from build123d import *

# Parameters (mm, degrees)
SKETCH_1_W          = 30
SKETCH_1_H          = 20
SKETCH_1_R          = 1.5
EXTRUDE_1_DEPTH     = 3
CUT_EXTRUDE_1_REACH = 20.276
SKETCH_2_R          = 2.5


with BuildPart() as part:
    # 草图1 → 凸台-拉伸1 (new body)
    with BuildSketch(Plane(origin=(0, 0, 0), x_dir=(0, 0, -1), z_dir=(1, 0, 0))):
        Rectangle(SKETCH_1_W, SKETCH_1_H)
        with Locations((-11, 6)):
            Circle(SKETCH_1_R, mode=Mode.SUBTRACT)
        with Locations((-11, -6)):
            Circle(SKETCH_1_R, mode=Mode.SUBTRACT)
        with Locations(Location((11, -6, 0), (0, 0, 180))):
            Circle(SKETCH_1_R, mode=Mode.SUBTRACT)
        with Locations(Location((11, 6, 0), (0, 0, 180))):
            Circle(SKETCH_1_R, mode=Mode.SUBTRACT)
    extrude(amount=EXTRUDE_1_DEPTH)

    # 草图2 → 切除-拉伸1 (cut, up to next)
    with BuildSketch(Plane.ZY, mode=Mode.PRIVATE) as cut_extrude_1_sk1:
        with Locations((0, -4)):
            Circle(SKETCH_2_R)
    cut_extrude_1_tool1 = extrude(cut_extrude_1_sk1.sketch, amount=-CUT_EXTRUDE_1_REACH, mode=Mode.PRIVATE) & part.part
    add(cut_extrude_1_tool1.solids().sort_by_distance((0, -4, 0))[0], mode=Mode.SUBTRACT)


solid = part.part
Source: CAD feature listing. Evaluate the final solid. Frame: model axes, mm. Give positions to 0.01 mm unless a question says otherwise; leave off trailing zeros. Loops run counter-clockwise (first coordinate to the right, second up) from the corner with the lowest first, then second, coordinate; pieces in that order, holes last. Notation, with made-up numbers: (81.5, -34.75) -> (112.5, -34.75) arc R26 cw to (112.5, -3.75) -> close; hole circle Ø6 at (-6.5, -37). An arc over 180 degrees is marked (long way). Use a Markdown table: item, result. Add a question column.
1) Section query A-A, the plane y = 6. Return the cut outline in (x, z).
2) Line query: line 1 along Y through (x, z) = (1.2, -11); line 2 along Z through (x, y) = (0.8, -6.25); line 3 along Z through (x, y) = (2.05, -5.25). Output: solid intervals per line, ascending. Write a range as [from, to].
3) Section query C-C, the plane z = -2. Return the cut outline in (x, y).
4) First-contact query: pin 1 (2.5 mm diameter, centred on y = -6, z = 11, fed in from +X). Flat tip, straight axial feed; report the tip coordinate or a pass-through.
5) Section query D-D, the plane y = -6. Return the cut outline in (x, z).
6) Section query B-B, the plane z = 11. Return the cut outline in (x, y), then the cut area to 3 significant figures.
7) Pull-direction query (Y, two-part tool) for faces 1 (the face through (1.48, -5.93, 12.5)), 2 (the face through (3, 0, 0)), 3 (the face through (1.48, -1.52, -0.33)), 4 (the face through (1, 10, 0)); classes: +Y half, -Y half, draft (parallel to the pull), parting line (faces both ways), or undercut.
Numbers:
| question | item | result |
|---|---|---|
| 1 | outline | (0, -15) -> (3, -15) -> (3, -12.5) -> (0, -12.5) -> close; (0, -9.5) -> (3, -9.5) -> (3, 9.5) -> (0, 9.5) -> close; (0, 12.5) -> (3, 12.5) -> (3, 15) -> (0, 15) -> close |
| 2 | line 1 | y = [-10, -7.5], [-4.5, 4.5], [7.5, 10] |
| 2 | line 2 | z = [-15, -12.48], [-9.52, -1.09], [1.09, 9.52], [12.48, 15] |
| 2 | line 3 | z = [-15, -12.3], [-9.7, -2.17], [2.17, 9.7], [12.3, 15] |
| 3 | outline | (0, -10) -> (3, -10) -> (3, -5.5) -> (0, -5.5) -> close; (0, -2.5) -> (3, -2.5) -> (3, 10) -> (0, 10) -> close |
| 4 | pin 1 | passes through |
| 5 | outline | (0, -15) -> (3, -15) -> (3, -12.5) -> (0, -12.5) -> close; (0, -9.5) -> (3, -9.5) -> (3, -1.5) -> (0, -1.5) -> close; (0, 1.5) -> (3, 1.5) -> (3, 9.5) -> (0, 9.5) -> close; (0, 12.5) -> (3, 12.5) -> (3, 15) -> (0, 15) -> close |
| 6 | outline | (0, -10) -> (3, -10) -> (3, -7.5) -> (0, -7.5) -> close; (0, -4.5) -> (3, -4.5) -> (3, 4.5) -> (0, 4.5) -> close; (0, 7.5) -> (3, 7.5) -> (3, 10) -> (0, 10) -> close |
| 6 | area | 42.0 mm2 |
| 7 | face 1 | undercut |
| 7 | face 2 | draft |
| 7 | face 3 | undercut |
| 7 | face 4 | +Y half |
